Can you work these out from the drawing? Everything is in mm from the part's minimum corner. A direction names the side the tool comes from. Give positions to 0.01 mm unless a question says otherwise; leave off trailing zeros. Loops run counter-clockwise (first coordinate to the right, second up) from the corner with the lowest first, then second, coordinate; pieces in that order, holes last. Notation, with made-up numbers: (50.5, 22) - (82.5, 22) arc R19 ccw to (82.5, 37) - close; hole circle Ø7 at (-20, 28.5). An arc over 180 degrees is marked (long way). Answer in a Markdown table with one row per item.
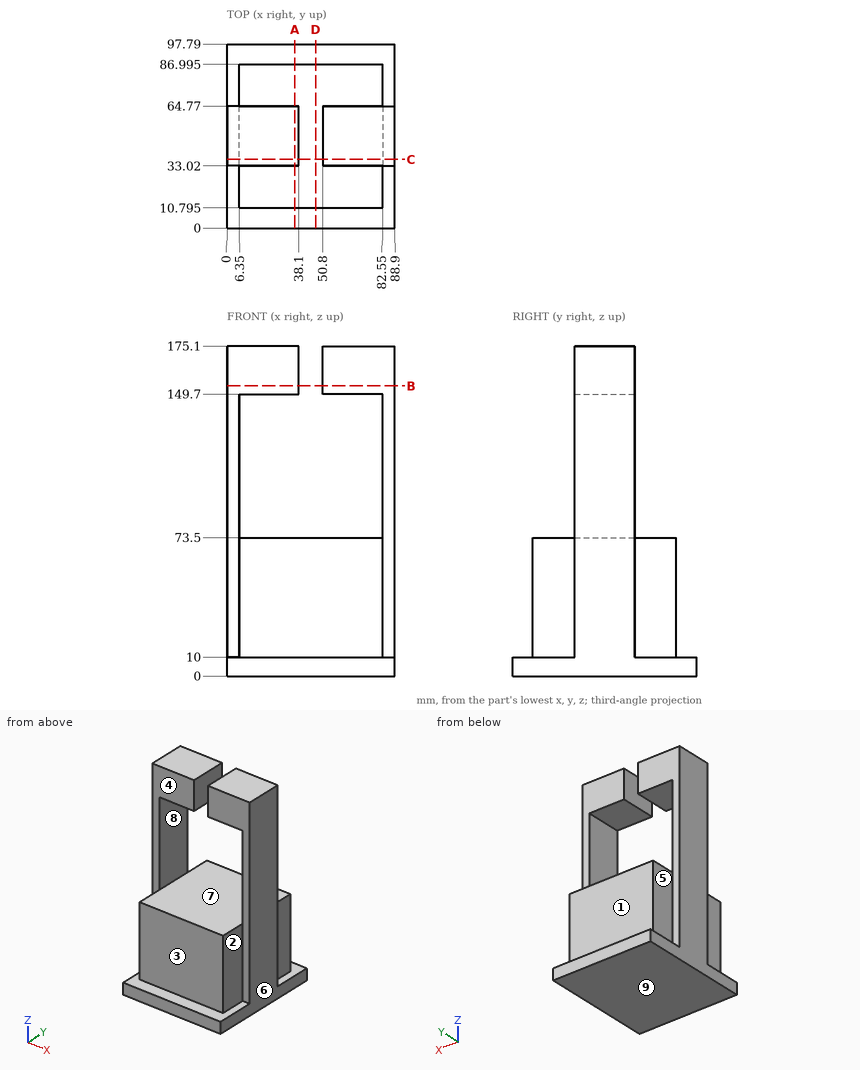
Q1. Imagine slicing it at D-D, the plane x = 47. Write out the boundary of the cut face in (y, z) (3 decimals), and give its area (3 significant figures).
Checked values:
| item | result |
|---|---|
| outline | (0, 0) - (97.79, 0) - (97.79, 10) - (86.995, 10) - (86.995, 73.5) - (10.795, 73.5) - (10.795, 10) - (0, 10) - close |
| area | 5,820 mm² |
Q2. Imagine slicing it at C-C, the plane y = 36.5. Write out the boundary of the cut face in (x, z), and give its area (3 significant figures).
Checked values:
| item | result |
|---|---|
| outline | (0, 0) - (88.9, 0) - (88.9, 175.1) - (50.8, 175.1) - (50.8, 149.7) - (82.55, 149.7) - (82.55, 73.5) - (6.35, 73.5) - (6.35, 149.7) - (38.1, 149.7) - (38.1, 175.1) - (0, 175.1) - close |
| area | 9,440 mm² |
Q3. If I drill on line 1 (Z direction, x = 17, y = 59); line 2 (X direction, y = 45, z = 144.5); line 3 (Y direction, x = 49, z = 58) (3 decimals), over which ranges is the centre line in solid material (lowest first)? Write a range as [from, to].
Checked values:
| item | result |
|---|---|
| line 1 | z = [0, 73.5], [149.7, 175.1] |
| line 2 | x = [0, 6.35], [82.55, 88.9] |
| line 3 | y = [10.795, 86.995] |
Q4. Imagine slicing it at B-B, the plane z = 154. Write out the boundary of the cut face in (x, y), and give its area (3 significant figures).
Checked values:
| item | result |
|---|---|
| outline | (0, 33.02) - (38.1, 33.02) - (38.1, 64.77) - (0, 64.77) - close; (50.8, 33.02) - (88.9, 33.02) - (88.9, 64.77) - (50.8, 64.77) - close |
| area | 2,420 mm² |
Q5. For pin 1 (2 mm diameter, centred on x = 40, y = 43.5, fed in from +Z); pin 2 (5 mm diameter, centred on x = 31.5, z = 51, fed in from -Y) (3 decimals); pin 3 (9.5 mm diameter, centred on y = 51.5, z = 129, fed in from -X); pin 4 (6.5 mm diameter, centred on y = 80, z = 54, fed in from -X), each with a flat end and sliding along its axis, tell me the tip position at first contact or that it passes through.
Checked values:
| item | result |
|---|---|
| pin 1 | stops at z = 73.5 |
| pin 2 | stops at y = 10.795 |
| pin 3 | stops at x = 0 |
| pin 4 | stops at x = 6.35 |
Q6. Imagine slicing it at A-A, the plane x = 36. Write out the boundary of the cut face in (y, z) (3 decimals).
Checked values:
| item | result |
|---|---|
| outline | (0, 0) - (97.79, 0) - (97.79, 10) - (86.995, 10) - (86.995, 73.5) - (10.795, 73.5) - (10.795, 10) - (0, 10) - close; (33.02, 149.7) - (64.77, 149.7) - (64.77, 175.1) - (33.02, 175.1) - close |
Q7. If we mould it in two halves opening along Z, with no side actions, what happens to the marked faces 6, 7, 8 and 9? For each: released by +Z, released by -Z, zero draft, split by the parting line, or undercut.
Checked values:
| item | result |
|---|---|
| face 6 | zero draft |
| face 7 | undercut |
| face 8 | undercut |
| face 9 | released by -Z |
Q8. On a 3-axis mill with a long thin cutter (end or side, diameter ignored), from which of +Z, -Z, +X, -X, +Y, -Y can I reach the whole of each face in a straight line? I mean the marked faces 1, 2, 3, 4 and 5. Say none if no direction works.
Checked values:
| item | result |
|---|---|
| face 1 | +Z, +X, -X, +Y |
| face 2 | +Z, +X, -Y |
| face 3 | +Z, +X, -X, -Y |
| face 4 | +Z, -X, -Y |
| face 5 | +Z, -X, +Y |
